Geometry: final body of the model. Coordinates: model frame, mm. A direction names the side the tool comes from. Give positions to 0.01 mm unless a question says otherwise; leave off trailing zeros. Loops run counter-clockwise (first coordinate to the right, second up) from the corner with the lowest first, then second, coordinate; pieces in that order, holes last.
from build123d import *

# Parameters (mm, degrees)
SKETCH1_W           = 48
SKETCH1_H           = 43
BOSS_EXTRUDE1_DEPTH = 5
CUT_EXTRUDE1_REACH  = 34.608
SKETCH2_R           = 1.55
SKETCH4_W           = 5
SKETCH4_H           = 43
BOSS_EXTRUDE2_DEPTH = 40
CUT_EXTRUDE2_REACH  = 71.219
SKETCH6_R           = 2
SKETCH7_R           = 3.5
CUT_EXTRUDE3_DEPTH  = 3


with BuildPart() as part:
    # Sketch1 → Boss-Extrude1 (new body)
    with BuildSketch(Plane(origin=(0, 0, 0), x_dir=(0, 0, -1), z_dir=(1, 0, 0))):
        Rectangle(SKETCH1_W, SKETCH1_H)
    extrude(amount=BOSS_EXTRUDE1_DEPTH)

    # Sketch2 → Cut-Extrude1 (cut, up to next)
    with BuildSketch(Plane(origin=(5, 0, 0), x_dir=(0, 0, -1), z_dir=(1, 0, 0)), mode=Mode.PRIVATE) as cut_extrude1_sk1:
        with Locations((-15.5, 15.5)):
            Circle(SKETCH2_R)
    cut_extrude1_tool1 = extrude(cut_extrude1_sk1.sketch, amount=-CUT_EXTRUDE1_REACH, mode=Mode.PRIVATE) & part.part
    # Sketch2 → Cut-Extrude1 (cut, up to next)
    with BuildSketch(Plane(origin=(5, 0, 0), x_dir=(0, 0, -1), z_dir=(1, 0, 0)), mode=Mode.PRIVATE) as cut_extrude1_sk2:
        with Locations((15.5, 15.5)):
            Circle(SKETCH2_R)
    cut_extrude1_tool2 = extrude(cut_extrude1_sk2.sketch, amount=-CUT_EXTRUDE1_REACH, mode=Mode.PRIVATE) & part.part
    # Sketch2 → Cut-Extrude1 (cut, up to next)
    with BuildSketch(Plane(origin=(5, 0, 0), x_dir=(0, 0, -1), z_dir=(1, 0, 0)), mode=Mode.PRIVATE) as cut_extrude1_sk3:
        with Locations((15.5, -15.5)):
            Circle(SKETCH2_R)
    cut_extrude1_tool3 = extrude(cut_extrude1_sk3.sketch, amount=-CUT_EXTRUDE1_REACH, mode=Mode.PRIVATE) & part.part
    # Sketch2 → Cut-Extrude1 (cut, up to next)
    with BuildSketch(Plane(origin=(5, 0, 0), x_dir=(0, 0, -1), z_dir=(1, 0, 0)), mode=Mode.PRIVATE) as cut_extrude1_sk4:
        with Locations((-15.5, -15.5)):
            Circle(SKETCH2_R)
    cut_extrude1_tool4 = extrude(cut_extrude1_sk4.sketch, amount=-CUT_EXTRUDE1_REACH, mode=Mode.PRIVATE) & part.part
    add(cut_extrude1_tool1.solids().sort_by_distance((5, 15.5, 15.5))[0], mode=Mode.SUBTRACT)
    add(cut_extrude1_tool2.solids().sort_by_distance((5, 15.5, -15.5))[0], mode=Mode.SUBTRACT)
    add(cut_extrude1_tool3.solids().sort_by_distance((5, -15.5, -15.5))[0], mode=Mode.SUBTRACT)
    add(cut_extrude1_tool4.solids().sort_by_distance((5, -15.5, 15.5))[0], mode=Mode.SUBTRACT)

    # Sketch4 → Boss-Extrude2 (add)
    with BuildSketch(Plane(origin=(5, 0, 0), x_dir=(0, 0, -1), z_dir=(1, 0, 0))):
        with Locations((-21.5, 0)):
            Rectangle(SKETCH4_W, SKETCH4_H)
    boss_extrude2 = extrude(amount=BOSS_EXTRUDE2_DEPTH)

    # Sketch6 → Cut-Extrude2 (cut, up to next)
    with BuildSketch(Plane.XY.offset(24), mode=Mode.PRIVATE) as cut_extrude2_sk1:
        with Locations((27, 12)):
            Circle(SKETCH6_R)
    cut_extrude2_tool1 = extrude(cut_extrude2_sk1.sketch, amount=-CUT_EXTRUDE2_REACH, mode=Mode.PRIVATE) & part.part
    # Sketch6 → Cut-Extrude2 (cut, up to next)
    with BuildSketch(Plane.XY.offset(24), mode=Mode.PRIVATE) as cut_extrude2_sk2:
        with Locations((39, 0)):
            Circle(SKETCH6_R)
    cut_extrude2_tool2 = extrude(cut_extrude2_sk2.sketch, amount=-CUT_EXTRUDE2_REACH, mode=Mode.PRIVATE) & part.part
    # Sketch6 → Cut-Extrude2 (cut, up to next)
    with BuildSketch(Plane.XY.offset(24), mode=Mode.PRIVATE) as cut_extrude2_sk3:
        with Locations((27, -12)):
            Circle(SKETCH6_R)
    cut_extrude2_tool3 = extrude(cut_extrude2_sk3.sketch, amount=-CUT_EXTRUDE2_REACH, mode=Mode.PRIVATE) & part.part
    # Sketch6 → Cut-Extrude2 (cut, up to next)
    with BuildSketch(Plane.XY.offset(24), mode=Mode.PRIVATE) as cut_extrude2_sk4:
        with Locations((15, 0)):
            Circle(SKETCH6_R)
    cut_extrude2_tool4 = extrude(cut_extrude2_sk4.sketch, amount=-CUT_EXTRUDE2_REACH, mode=Mode.PRIVATE) & part.part
    cut_extrude2_1 = cut_extrude2_tool1.solids().sort_by_distance((27, 12, 24))[0]
    add(cut_extrude2_1, mode=Mode.SUBTRACT)
    cut_extrude2_2 = cut_extrude2_tool2.solids().sort_by_distance((39, 0, 24))[0]
    add(cut_extrude2_2, mode=Mode.SUBTRACT)
    cut_extrude2_3 = cut_extrude2_tool3.solids().sort_by_distance((27, -12, 24))[0]
    add(cut_extrude2_3, mode=Mode.SUBTRACT)
    cut_extrude2_4 = cut_extrude2_tool4.solids().sort_by_distance((15, 0, 24))[0]
    add(cut_extrude2_4, mode=Mode.SUBTRACT)
    cut_extrude2 = cut_extrude2_1 + cut_extrude2_2 + cut_extrude2_3 + cut_extrude2_4  # Cut-Extrude2 as one shape, for the pattern or mirror that repeats it

    # Sketch7 → Cut-Extrude3 (cut)
    with BuildSketch(Plane.XY.offset(24)):
        with Locations((27, 12)):
            Circle(SKETCH7_R)
        with Locations((39, 0)):
            Circle(SKETCH7_R)
        with Locations((27, -12)):
            Circle(SKETCH7_R)
        with Locations((15, 0)):
            Circle(SKETCH7_R)
    cut_extrude3 = extrude(amount=-CUT_EXTRUDE3_DEPTH, mode=Mode.SUBTRACT)

    # Mirror2: Boss-Extrude2, Cut-Extrude2, Cut-Extrude3 across plane
    add(boss_extrude2.mirror(Plane.XY))
    add(cut_extrude2.mirror(Plane.XY), mode=Mode.SUBTRACT)
    add(cut_extrude3.mirror(Plane.XY), mode=Mode.SUBTRACT)


solid = part.part
Item 1: Draft query along X for faces 1 (the face through (41, -2, -21)), 2 (the face through (45, 0, 22)), 3 (the face through (2.54, -14.45, 16.64)). Return one class per face: +X half, -X half, draft (parallel to the pull), parting line (faces both ways), or undercut.
Values follow:
face 1: undercut
face 2: +X half
face 3: draft
Item 2: Section query D-D on y = 0. Give the number of separate pieces and of enclosed holes in the cut face, plus the area to 3 significant figures.
Values follow:
separate pieces: 5
enclosed holes: 0
area: 524 mm2
Item 3: Set-up query: faces 4 (the face through (5, 0, 0)), 5 (the face through (28.615, 8.895, 22.521)), 6 (the face through (35.503, 0.154, -22.521)). Return all of +Z, -Z, +X, -X, +Y, -Y with unobstructed straight access to the full face (end or side cutting, diameter ignored); none if empty.
Values follow:
face 4: +X, +Y, -Y
face 5: +Z
face 6: -Z
Item 4: Section query A-A on x = 34. Return loops of the section in (y, z), plus the area to 3 significant figures.
Values follow:
outline: (-21.5, -24) - (21.5, -24) - (21.5, -19) - (-21.5, -19) - close; (-21.5, 19) - (21.5, 19) - (21.5, 24) - (-21.5, 24) - close
area: 430 mm2
Item 5: Pin query (flat end, axial travel): pin 1 (4.5 mm diameter, centred on x = 39, y = 0, fed in from -Z); pin 2 (5 mm diameter, centred on y = 2.5, z = 5.5, fed in from +X); pin 3 (3 mm diameter, centred on x = 27, y = -12, fed in from +Z); pin 4 (2 mm diameter, centred on x = 40.5, y = 1.5, fed in from +Z). Return the tip coordinate at first contact, or that it passes through.
Values follow:
pin 1: stops at z = -21
pin 2: stops at x = 5
pin 3: passes through
pin 4: stops at z = 21
Item 6: Ray query, probe 1 along Y at (x, z) = (27, -20); probe 2 along Y at (x, z) = (2.65, -15.5); probe 3 along Z at (x, y) = (18.5, 2.5). Return the intervals inside material, ascending.
Values follow:
probe 1: y = -21.5 to -14, -10 to 10, 14 to 21.5
probe 2: y = -21.5 to -17.05, -13.95 to 13.95, 17.05 to 21.5
probe 3: z = -24 to -19, 19 to 24
Item 7: Section query C-C on y = 6.5. Return loops of the section in (x, z), plus the area to 3 significant figures.
Values follow:
outline: (0, -24) - (45, -24) - (45, -19) - (5, -19) - (5, 19) - (45, 19) - (45, 24) - (0, 24) - close
area: 640 mm2
Item 8: Section query B-B on z = -15.5. Return loops of the section in (x, y), plus the area to 3 significant figures.
Values follow:
outline: (0, -21.5) - (5, -21.5) - (5, -17.05) - (0, -17.05) - close; (0, -13.95) - (5, -13.95) - (5, 13.95) - (0, 13.95) - close; (0, 17.05) - (5, 17.05) - (5, 21.5) - (0, 21.5) - close
area: 184 mm2
